The listing builds one solid part. Answer for the finished solid, in the listing's coordinates (mm). A direction names the side the tool comes from. Give positions to 0.01 mm unless a question says otherwise; leave off trailing zeros. Write each loop counter-clockwise with the first axis right and the second up, starting at its lowest first coordinate (ties: lowest second). Pieces come first, ordered by that corner, then holes. Notation, with made-up numbers: (46.5, 8) - (92.5, 8) arc R31 cw to (92.5, 38) - close; hole circle Ø3 at (-23, 40.25). An arc over 180 degrees is marked (long way). Answer as CSV lines item,"result". Start each with the question number.
(1) For a pull along X with two mould halves and no side action, classify faces 3 (the face through (-66.63, -28.62, 3.13)), 4 (the face through (-9.525, 24, 3)), 5 (the face through (-1, 31.75, 3)) as pulls with the +X half, pulls with the -X half, needs draft (parallel to the pull), parting line crosses it, or undercut.
(2) Find section A-A (x = 25). Write down the section's boundary in (y, z) (3 decimals).
(3) Straight lines are drawn through the part: probe 1 along X at (y, z) = (-8.5, 3); probe 2 along Y at (x, z) = (25, 1.75) (3 decimals); probe 3 along X at (y, z) = (28, 6). For each, find the intervals that lie inside material, in ascending order.
(4) For faces 1 (the face through (-17, 22, 6.35)), 2 (the face through (35, 20.955, 3)), determine the directions among +Z, -Z, +X, -X, +Y, -Y from which every point of the face is accessible in a straight line to the end or side of a thin tool.
(5) Find section C-C (z = 2). State how many separate pieces and enclosed holes the cut face has, then the cut area to 3 significant figures.
(6) Find section B-B (y = -0.5). Write down the section's boundary in (x, z).
from build123d import *

# Parameters (mm, degrees)
F0_W     = 139.7
F0_H     = 63.5
F0_R     = 1.7145
F0_R_2   = 1.0922
F1_DEPTH = 6.35
F2_SIZE  = 6.35


with BuildPart() as f1:
    # F0 (on Top) → F1 (new body)
    with BuildSketch(Plane.XY):
        Rectangle(F0_W, F0_H)
        with Locations((-57.404, -27.178)):
            Circle(F0_R, mode=Mode.SUBTRACT)
        with Locations((-56.261, -22.86)):
            Circle(F0_R_2, mode=Mode.SUBTRACT)
        with Locations((57.404, -27.178)):
            Circle(F0_R, mode=Mode.SUBTRACT)
        with Locations((56.261, -22.86)):
            Circle(F0_R_2, mode=Mode.SUBTRACT)
        with Locations((-56.261, 22.86)):
            Circle(F0_R_2, mode=Mode.SUBTRACT)
        with Locations((-57.404, 27.178)):
            Circle(F0_R, mode=Mode.SUBTRACT)
        Polygon((9.525, 20.955), (60.452, 20.955), (60.452, -20.955), (-60.452, -20.955), (-60.452, 20.955), (-9.525, 20.955), (-9.525, 27.305), (9.525, 27.305), align=None, mode=Mode.SUBTRACT)
        with Locations((56.261, 22.86)):
            Circle(F0_R_2, mode=Mode.SUBTRACT)
        with Locations((57.404, 27.178)):
            Circle(F0_R, mode=Mode.SUBTRACT)
    extrude(amount=F1_DEPTH)

    # F2
    f2_edges = [f1.edges().sort_by_distance(p)[0] for p in [
        (-69.85, -31.75, 3.175),
        (69.85, 31.75, 3.175),
        (-69.85, 31.75, 3.175),
        (69.85, -31.75, 3.175),
    ]]
    chamfer(f2_edges, length=F2_SIZE)


solid = f1.part
Result set:
1,face 3,"pulls with the -X half"
1,face 4,"undercut"
1,face 5,"needs draft"
2,outline,"(-31.75, 0) - (-20.955, 0) - (-20.955, 6.35) - (-31.75, 6.35) - close; (20.955, 0) - (31.75, 0) - (31.75, 6.35) - (20.955, 6.35) - close"
3,probe 1,"-69.85 to -60.45, 60.45 to 69.85"
3,probe 2,"-31.75 to -20.955, 20.955 to 31.75"
3,probe 3,"-67.25 to -58.91, -55.9 to 55.9, 58.91 to 67.25"
4,face 1,"+Z, +X, -X, +Y, -Y"
4,face 2,"+Z, -Z"
5,separate pieces,"1"
5,enclosed holes,"9"
5,area,"3,550 mm^2"
6,outline,"(-69.85, 0) - (-60.45, 0) - (-60.45, 6.35) - (-69.85, 6.35) - close; (60.45, 0) - (69.85, 0) - (69.85, 6.35) - (60.45, 6.35) - close"
